For this review, take the finished solid that the model builds, in its own axes (mm). Face numbers are marked on the shaded views. A direction names the side the tool comes from. Coordinates: 2 decimals unless noted, no trailing zeros. Loops run counter-clockwise (first coordinate to the right, second up) from the corner with the lowest first, then second, coordinate; pieces in that order, holes last.
1. Machinability: for the marked faces 1 and 2, which of the approach directions +Z, -Z, +X, -X, +Y, -Y give a long, thin tool a straight path to every point of the face, cutting with its end or side? Answer none if there is none.
2. Clearance check with flat-ended pins moving along their axes: P1, Ø3.5, axis at x = 6.5, y = 21, coming from the -Z side; P2, Ø10, axis at y = 19.5, z = 24, coming from the -X side; P3, Ø2.5, axis at y = 20.5, z = -54.5, coming from the +X side; P4, Ø3, axis at x = 33.5, y = 18, coming from the -Z side. State where each tip first meets the part, or that it passes through.
3. To check wall thickness, follow probe 1 along Z at (x, y) = (27, 14.5); probe 2 along Y at (x, z) = (46, -23); probe 3 along Y at (x, z) = (5.5, 23). State the ranges of each line that lie inside material, in increasing order.
4. Take a section at C-C, the plane x = 6.25. State the section outline as (y, z) points (3 decimals).
5. Take a section at D-D, the plane x = 16. State the section outline as (y, z) points.
6. Take a section at A-A, the plane z = -51. State the section outline as (x, y) points, then the cut area to 3 significant figures.
7. Take a section at B-B, the plane y = 3.5. State the section outline as (x, z) points, then the cut area to 3 significant figures.
```python
from build123d import *

# Parameters (mm, degrees)
SKETCH1_W           = 64.5
SKETCH1_H           = 19.5
BOSS_EXTRUDE1_DEPTH = 69
FILLET1_R           = 2
FILLET2_R           = 2
SKETCH2_R           = 2.875
BOSS_EXTRUDE2_DEPTH = 35
SKETCH3_W           = 3.5
SKETCH3_H           = 7
BOSS_EXTRUDE3_DEPTH = 3


with BuildPart() as part:
    # Sketch1 → Boss-Extrude1 (new body)
    with BuildSketch(Plane(origin=(0, 0, 0), x_dir=(0, 0, -1), z_dir=(1, 0, 0))):
        with Locations((32.25, 9.75)):
            Rectangle(SKETCH1_W, SKETCH1_H)
    extrude(amount=BOSS_EXTRUDE1_DEPTH)

    # Fillet1
    fillet1_edges = [part.edges().sort_by_distance(p)[0] for p in [
        (34.5, 19.5, 0),
        (34.5, 19.5, -64.5),
        (34.5, 0, -64.5),
        (34.5, 0, 0),
    ]]
    fillet(fillet1_edges, radius=FILLET1_R)

    # Fillet2
    fillet2_edges = [part.edges().sort_by_distance(p)[0] for p in [
        (0, 0, -32.25),
        (69, 0, -32.25),
        (0, 9.75, 0),
        (0, 19.5, -32.25),
        (0, 9.75, -64.5),
        (0, 18.914213562, -63.914213562),
        (0, 0.585786438, -63.914213562),
        (0, 18.914213562, -0.585786438),
        (0, 0.585786438, -0.585786438),
        (69, 9.75, 0),
        (69, 9.75, -64.5),
        (69, 19.5, -32.25),
        (69, 18.914213562, -63.914213562),
        (69, 0.585786438, -63.914213562),
        (69, 18.914213562, -0.585786438),
        (69, 0.585786438, -0.585786438),
    ]]
    fillet(fillet2_edges, radius=FILLET2_R)

    # Sketch2 → Boss-Extrude2 (add)
    with BuildSketch(Plane.XY):
        with Locations(Location((6.25, 13.5, 0), (0, 0, 180))):
            Circle(SKETCH2_R)
    extrude(amount=BOSS_EXTRUDE2_DEPTH)

    # Sketch3 → Boss-Extrude3 (add)
    with BuildSketch(Plane(origin=(0, 19.5, 0), x_dir=(1, 0, 0), z_dir=(0, 1, 0))):
        with Locations((6.75, 53)):
            Rectangle(SKETCH3_W, SKETCH3_H)
    extrude(amount=BOSS_EXTRUDE3_DEPTH)


solid = part.part
```
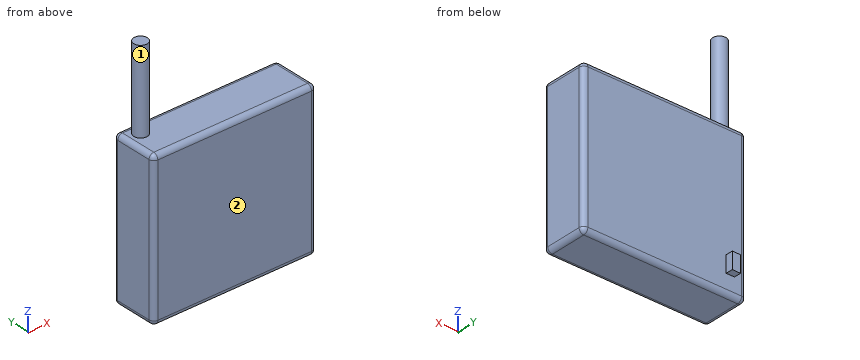
Results list:
1. face 1: +Z
1. face 2: +Z, -Z, +X, -X, -Y
2. P1: stops at z = -63.47
2. P2: stops at x = 3.55
2. P3: stops at x = 67.97
2. P4: stops at z = -64.5
3. probe 1: z = -64.5 to 0
3. probe 2: y = 0 to 19.5
3. probe 3: y = 10.72 to 16.28
4. outline: (0, -62.5) arc R2 ccw to (2, -64.5) - (17.5, -64.5) arc R2 ccw to (19.5, -62.5) - (19.5, -56.5) - (22.5, -56.5) - (22.5, -49.5) - (19.5, -49.5) - (19.5, -2) arc R2 ccw to (17.5, 0) - (16.375, 0) - (16.375, 35) - (10.625, 35) - (10.625, 0) - (2, 0) arc R2 ccw to (0, -2) - close
5. outline: (0, -62.5) arc R2 ccw to (2, -64.5) - (17.5, -64.5) arc R2 ccw to (19.5, -62.5) - (19.5, -2) arc R2 ccw to (17.5, 0) - (2, 0) arc R2 ccw to (0, -2) - close
6. outline: (0, 2) arc R2 ccw to (2, 0) - (67, 0) arc R2 ccw to (69, 2) - (69, 17.5) arc R2 ccw to (67, 19.5) - (8.5, 19.5) - (8.5, 22.5) - (5, 22.5) - (5, 19.5) - (2, 19.5) arc R2 ccw to (0, 17.5) - close
6. area: 1,350 mm2
7. outline: (0, -62.5) arc R2 ccw to (2, -64.5) - (67, -64.5) arc R2 ccw to (69, -62.5) - (69, -2) arc R2 ccw to (67, 0) - (2, 0) arc R2 ccw to (0, -2) - close
7. area: 4,450 mm2
